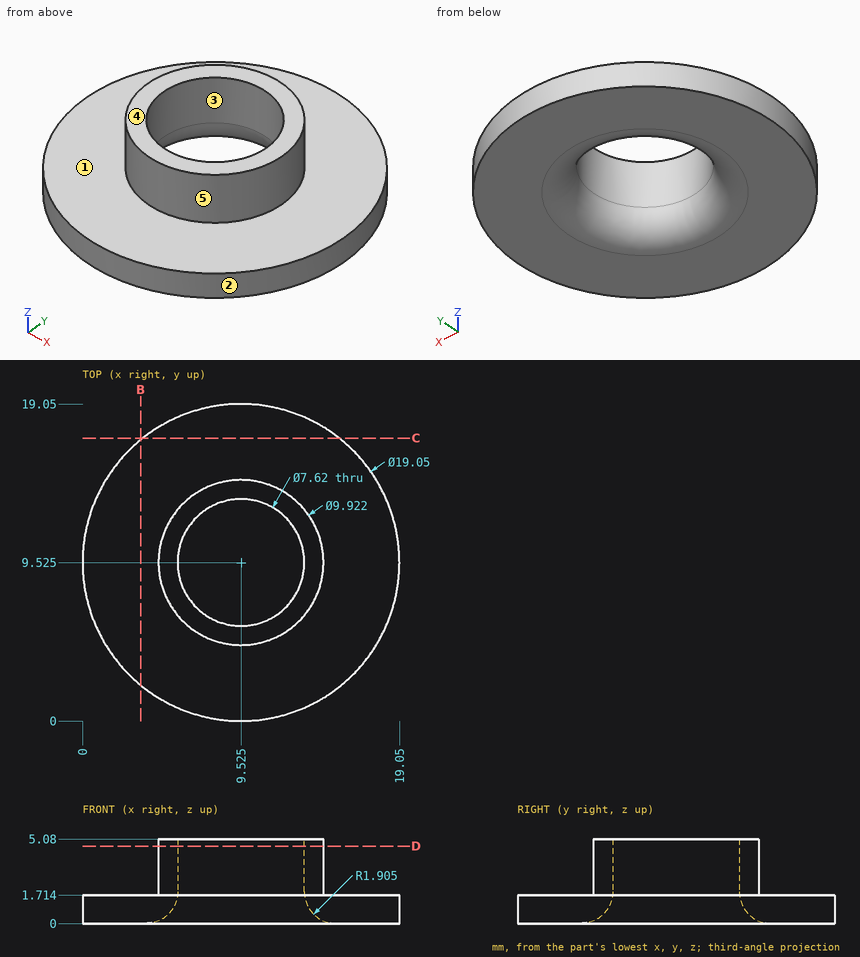
Can you work these out from the drawing? Everything is in mm from the part's minimum corner. A direction names the side the tool comes from. Give positions to 0.01 mm unless a question says otherwise; leave off trailing zeros. Loops run counter-clockwise (first coordinate to the right, second up) from the corner with the lowest first, then second, coordinate; pieces in that order, holes last. Notation, with made-up numbers: (-19.75, 36.5) -> (-9.75, 36.5) arc R25 ccw to (-9.75, 61.5) -> close; hole circle Ø6 at (-4, 6). An arc over 180 degrees is marked (long way). Return JSON: item names as keys, results as strings.
Item 1: If we section it at C-C on y = 17: List the corners of the cut face in (x, z) for me (1 decimal).
Geometry results:
{"outline": "(3.6, 0) -> (15.4, 0) -> (15.4, 1.7) -> (3.6, 1.7) -> close"}
Item 2: I'm going to push flat-ended pins straight in: pin 1 (1 mm diameter, centred on x = 3.5, z = 1.5, fed in from +Y) (1 decimal); pin 2 (2 mm diameter, centred on y = 16, z = 2, fed in from +X); pin 3 (4 mm diameter, centred on x = 12, y = 9, fed in from -Z) (1 decimal). Where does each tip first touch, or does it pass through?
Geometry results:
{"pin 1": "stops at y = 17.3", "pin 2": "stops at x = 17.29", "pin 3": "stops at z = 0.4"}
Item 3: We'd pull the mould along Y, two halves only. Please class the marked faces 3, 4 and 5: +Y half, -Y half, draft (parallel to the pull), parting line (faces both ways), or undercut.
Geometry results:
{"face 3": "undercut", "face 4": "draft", "face 5": "parting line"}
Item 4: If we section it at B-B on x = 3.5: List the corners of the cut face in (y, z) for me (1 decimal).
Geometry results:
{"outline": "(2.1, 0) -> (16.9, 0) -> (16.9, 1.7) -> (2.1, 1.7) -> close"}
Item 5: I need wall thicknesses on L1, parallel to X at y = 9.5, z = 2.35 (1 decimal); L2, parallel to Z at x = 5.5, y = 17.5 (1 decimal); L3, parallel to X at y = 11.75, z = 3.5. Which ranges of each line are inside material? Lowest first, please. Write a range as from..to.
Geometry results:
{"L1": "x = 4.6..5.7, 13.3..14.5", "L2": "z = 0..1.7", "L3": "x = 5.09..6.43, 12.62..13.96"}
Item 6: If we section it at D-D on z = 4.65: List the corners of the cut face in (x, y) for me (1 decimal).
Geometry results:
{"outline": "circle Ø9.9 at (9.5, 9.5); hole circle Ø7.6 at (9.5, 9.5)"}
Item 7: Which directions (+Z, -Z, +X, -X, +Y, -Y) give clear straight access to the entire face, cutting with the end or side of a thin tool? Please do the marked faces 1 and 2.
Geometry results:
{"face 1": "+Z", "face 2": "+Z, -Z"}
